Read the model definition and answer for the solid it produces. Units are mm, in the model's axes. Face numbers are marked on the shaded views. Round coordinates to 2 decimals unless told otherwise and drop trailing zeros. Order: outer loops, then holes, each group sorted by start corner. A loop starts at its lowest first (then second) coordinate and runs counter-clockwise, first axis right, second up.
from build123d import *

# Parameters (mm, degrees)
SKETCH1_R          = 3
SKETCH1_R_2        = 1.5
EXTRUDE1_DEPTH     = 10
SKETCH2_R          = 5
CUT_EXTRUDE1_DEPTH = 6
SKETCH3_R          = 18
CUT_EXTRUDE2_DEPTH = 20


with BuildPart() as part:
    # Sketch1 → Extrude1 (new body)
    with BuildSketch(Plane.XY):
        Polygon((5, 135), (0, 135), (-24, 135), (-34, 135), (-34, 0), (-24, 0), (0, 0), (40, 0), (64, 0), (74, 0), (74, 135), (64, 135), (40, 135), align=None)
        with Locations((-25, 22.5)):
            Circle(SKETCH1_R, mode=Mode.SUBTRACT)
        with Locations((5, 22.5)):
            Circle(SKETCH1_R, mode=Mode.SUBTRACT)
        with Locations((-5, 42.5)):
            Circle(SKETCH1_R_2, mode=Mode.SUBTRACT)
        with Locations((35, 22.5)):
            Circle(SKETCH1_R, mode=Mode.SUBTRACT)
        with Locations((65, 22.5)):
            Circle(SKETCH1_R, mode=Mode.SUBTRACT)
        with Locations((45, 42.5)):
            Circle(SKETCH1_R_2, mode=Mode.SUBTRACT)
        with Locations((-25, 67.5)):
            Circle(SKETCH1_R, mode=Mode.SUBTRACT)
        with Locations((-5, 92.5)):
            Circle(SKETCH1_R_2, mode=Mode.SUBTRACT)
        with Locations((-25, 112.5)):
            Circle(SKETCH1_R, mode=Mode.SUBTRACT)
        with Locations((5, 112.5)):
            Circle(SKETCH1_R, mode=Mode.SUBTRACT)
        with Locations((45, 92.5)):
            Circle(SKETCH1_R_2, mode=Mode.SUBTRACT)
        with Locations((65, 67.5)):
            Circle(SKETCH1_R, mode=Mode.SUBTRACT)
        with Locations((35, 112.5)):
            Circle(SKETCH1_R, mode=Mode.SUBTRACT)
        with Locations((65, 112.5)):
            Circle(SKETCH1_R, mode=Mode.SUBTRACT)
    extrude(amount=EXTRUDE1_DEPTH)

    # Sketch2 → Cut-Extrude1 (cut)
    with BuildSketch(Plane(origin=(0, 0, 0), x_dir=(-1, 0, 0), z_dir=(0, 0, -1))):
        with Locations((-35, 112.5)):
            Circle(SKETCH2_R)
        with Locations((-65, 112.5)):
            Circle(SKETCH2_R)
        with Locations((-65, 22.5)):
            Circle(SKETCH2_R)
        with Locations((-5, 112.5)):
            Circle(SKETCH2_R)
        with Locations((-35, 22.5)):
            Circle(SKETCH2_R)
        with Locations((25, 22.5)):
            Circle(SKETCH2_R)
        with Locations((25, 112.5)):
            Circle(SKETCH2_R)
        with Locations((-5, 22.5)):
            Circle(SKETCH2_R)
        with Locations((-65, 67.5)):
            Circle(SKETCH2_R)
        with Locations((25, 67.5)):
            Circle(SKETCH2_R)
    extrude(amount=-CUT_EXTRUDE1_DEPTH, mode=Mode.SUBTRACT)

    # Sketch3 → Cut-Extrude2 (cut)
    with BuildSketch(Plane(origin=(0, 0, 0), x_dir=(-1, 0, 0), z_dir=(0, 0, -1))):
        with Locations((-20, 67.5)):
            Circle(SKETCH3_R)
    extrude(amount=-CUT_EXTRUDE2_DEPTH, mode=Mode.SUBTRACT)


solid = part.part
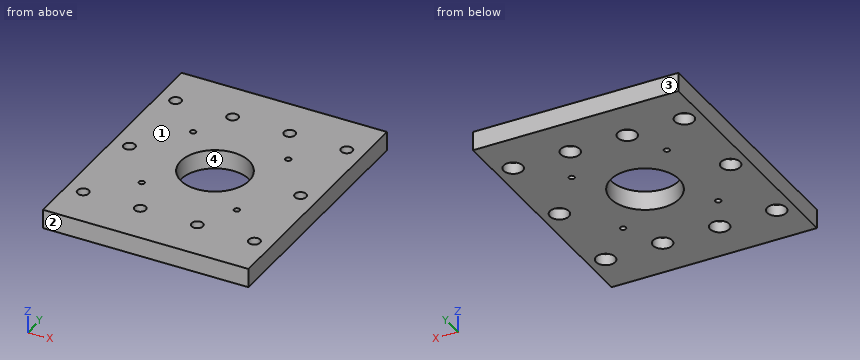
Q1. A cutting plane is placed at D-D, the plane x = -25. Give the vertices of the cut face in (y, z).
Outcome:
outline: (0, 0) - (17.5, 0) - (17.5, 6) - (19.5, 6) - (19.5, 10) - (0, 10) - close; (25.5, 6) - (27.5, 6) - (27.5, 0) - (62.5, 0) - (62.5, 6) - (64.5, 6) - (64.5, 10) - (25.5, 10) - close; (70.5, 6) - (72.5, 6) - (72.5, 0) - (107.5, 0) - (107.5, 6) - (109.5, 6) - (109.5, 10) - (70.5, 10) - close; (115.5, 6) - (117.5, 6) - (117.5, 0) - (135, 0) - (135, 10) - (115.5, 10) - close
Q2. A cutting plane is placed at C-C, the plane z = 8.25. Give the number of separate pieces and of enclosed holes in the cut face, plus the area to 3 significant figures.
Outcome:
separate pieces: 1
enclosed holes: 15
area: 13,300 mm2
Q3. A flat-ended cylindrical pin translates along its axis: pin 1 (3 mm diameter, centred on x = -25.5, y = 114, fed in from -Z). Find the tip coordinate at first contact, or state that the pin passes through.
Outcome:
pin 1: stops at z = 6
Q4. For a pull along Y with two mould halves and no side action, classify the marked faces 1, 2, 3 and 4 as released by +Y, released by -Y, zero draft, split by the parting line, or undercut.
Outcome:
face 1: zero draft
face 2: released by -Y
face 3: released by +Y
face 4: undercut
Q5. Straight lines are drawn through the part: probe 1 along Y at (x, z) = (-25, 7.6); probe 2 along X at (y, z) = (112.5, 8.1); probe 3 along Y at (x, z) = (-25, 4.7). For each, find the intervals that lie inside material, in ascending order.
Outcome:
probe 1: y = 0 to 19.5, 25.5 to 64.5, 70.5 to 109.5, 115.5 to 135
probe 2: x = -34 to -28, -22 to 2, 8 to 32, 38 to 62, 68 to 74
probe 3: y = 0 to 17.5, 27.5 to 62.5, 72.5 to 107.5, 117.5 to 135
Q6. A cutting plane is placed at B-B, the plane x = -5. Give the vertices of the cut face in (y, z).
Outcome:
outline: (0, 0) - (41, 0) - (41, 10) - (0, 10) - close; (44, 0) - (91, 0) - (91, 10) - (44, 10) - close; (94, 0) - (135, 0) - (135, 10) - (94, 10) - close
Q7. A cutting plane is placed at A-A, the plane y = 92.5. Give the vertices of the cut face in (x, z).
Outcome:
outline: (-34, 0) - (-6.5, 0) - (-6.5, 10) - (-34, 10) - close; (-3.5, 0) - (43.5, 0) - (43.5, 10) - (-3.5, 10) - close; (46.5, 0) - (74, 0) - (74, 10) - (46.5, 10) - close
